from build123d import *

# Parameters (mm, degrees)
SKETCH_1_W      = 4
SKETCH_1_H      = 1
SKETCH_1_W_2    = 1
SKETCH_1_H_2    = 4
EXTRUDE_1_DEPTH = 8
CHAMFER_1_SIZE  = 0.5
CHAMFER_2_SIZE  = 0.5
SKETCH_2_R      = 7.5
EXTRUDE_2_DEPTH = 2
FILLET_1_R      = 1


# Some blends are built 0.0001 mm under size
with BuildPart() as part:
    # 草图1 → 凸台-拉伸1 (new body)
    with BuildSketch(Plane.XY):
        Rectangle(SKETCH_1_W, SKETCH_1_H)
        Rectangle(SKETCH_1_W_2, SKETCH_1_H_2)
    extrude(amount=EXTRUDE_1_DEPTH)

    # 倒角1
    chamfer_1_edges = [part.edges().sort_by_distance(p)[0] for p in [
        (-1.25, -0.5, 8),
        (-0.5, -1.25, 8),
        (0.5, -1.25, 8),
        (1.25, -0.5, 8),
        (-1.25, 0.5, 8),
        (-0.5, 1.25, 8),
        (1.25, 0.5, 8),
        (0.5, 1.25, 8),
    ]]
    chamfer(chamfer_1_edges, length=CHAMFER_1_SIZE - 0.0001)  # a hair under: the kernel refuses the full size

    # 倒角2
    # the kernel refuses this chamfer: 0.5 mm, written as the material it takes off along each edge
    with BuildSketch(Plane(origin=(-2, 1.40922724, 6.59087276), x_dir=(0.9996219169112968, 0.01944252080601401, 0.019442520806014003), z_dir=(0, -0.7071067811865474, 0.7071067811865477)), Plane(origin=(0.90912724, -2, 8.90922724), x_dir=(0.7068394360706737, -0.02749587661058652, -0.7068394360706732), z_dir=(-0.7071067811865474, 0, -0.7071067811865477)), Plane(origin=(2, 0.90912724, 8.90922724), x_dir=(0.027495876610586514, 0.7068394360706736, -0.7068394360706733), z_dir=(0, -0.7071067811865474, -0.7071067811865477)), Plane(origin=(-0.90912724, 2, 8.90922724), x_dir=(-0.7068394360706737, 0.02749587661058652, -0.7068394360706732), z_dir=(0.7071067811865474, 0, -0.7071067811865477)), Plane(origin=(-1.40922724, 2, 6.59087276), x_dir=(0.7068394360706737, 0.027495876610586494, -0.7068394360706733), z_dir=(0.7071067811865474, 0, 0.7071067811865477))) as chamfer_2_piece_1:
        Polygon((CHAMFER_2_SIZE * 0.999621916911, -CHAMFER_2_SIZE * 0.0274958766106), (-CHAMFER_2_SIZE * 0.0274958766106, -CHAMFER_2_SIZE * 0.999621916911), (0, 0), align=None)
    extrude(amount=3.278648348, mode=Mode.SUBTRACT)
    with BuildSketch(Plane(origin=(-2, 0.90912724, 8.90922724), x_dir=(-0.027495876610586514, 0.7068394360706736, -0.7068394360706733), z_dir=(0, -0.7071067811865474, -0.7071067811865477)), Plane(origin=(-0.90912724, -2, 8.90922724), x_dir=(-0.7068394360706737, -0.02749587661058652, -0.7068394360706732), z_dir=(0.7071067811865474, 0, -0.7071067811865477)), Plane(origin=(2, -0.90912724, 8.90922724), x_dir=(0.027495876610586514, -0.7068394360706736, -0.7068394360706733), z_dir=(0, 0.7071067811865474, -0.7071067811865477))) as chamfer_2_piece_2:
        Polygon((CHAMFER_2_SIZE * 0.999621916911, CHAMFER_2_SIZE * 0.0274958766106), (-CHAMFER_2_SIZE * 0.0274958766106, CHAMFER_2_SIZE * 0.999621916911), (0, 0), align=None)
    extrude(amount=3.278648348, mode=Mode.SUBTRACT)

    # 草图2 → 凸台-拉伸2 (add)
    with BuildSketch(Plane(origin=(0, 0, 0), x_dir=(-1, 0, 0), z_dir=(0, 0, -1))):
        Circle(SKETCH_2_R)
    extrude(amount=EXTRUDE_2_DEPTH)

    # 圆角1
    fillet_1_edges = [part.edges().sort_by_distance(p)[0] for p in [
        (7.5, 0, 0),
        (7.5, 0, -2),
    ]]
    fillet(fillet_1_edges, radius=FILLET_1_R - 0.0001)  # a hair under: the kernel refuses the full size


solid = part.part
CAD build for the part. Positions are in the model's coordinates, mm. A direction names the side the tool comes from. Round coordinates to 2 decimals unless told otherwise and drop trailing zeros. Order: outer loops, then holes, each group sorted by start corner. A loop starts at its lowest first (then second) coordinate and runs counter-clockwise, first axis right, second up. Notation, with made-up numbers: (71, -28) -> (114, -28) arc R30 ccw to (114, 3) -> close; hole circle Ø10 at (0.25, 66). An arc over 180 degrees is marked (long way). Write each question's results on one line, items separated by ' | '.
1. Cut at A-A (z = 2.75). Give the cut face in (x, y), plus the area to 3 significant figures.
Findings below:
outline: (-2, -0.5) -> (-0.5, -0.5) -> (-0.5, -2) -> (0.5, -2) -> (0.5, -0.5) -> (2, -0.5) -> (2, 0.5) -> (0.5, 0.5) -> (0.5, 2) -> (-0.5, 2) -> (-0.5, 0.5) -> (-2, 0.5) -> close | area: 7.00 mm²
2. 3-axis set-ups, long thin cutter, end or side, ignore diameter. For faces 1 (the face through (2, 0, 4)), 2 (the face through (0, -2, 4)), 3 (the face through (0, 2, 4)), 4 (the face through (-0.5, -1, 4)), 5 (the face through (1, 0.5, 4)): which of +Z, -Z, +X, -X, +Y, -Y reach the whole face in a straight line?
Findings below:
face 1: +Z, +X, +Y, -Y | face 2: +Z, +X, -X, -Y | face 3: +Z, +X, -X, +Y | face 4: +Z, -X, -Y | face 5: +Z, +X, +Y
3. Wall check: line 1 along Z through (x, y) = (-1, 5); line 2 along X through (y, z) = (-1.75, 6). Give the ranges that are in metal, low to high. Write a range as [from, to].
Findings below:
line 1: z = [-2, 0] | line 2: x = [-0.5, 0.5]
4. Flat gauge pins, fed straight in: P1, Ø1.5, axis at x = -5, y = -1, coming from the +Z side; P2, Ø0.8, axis at y = 1, z = 3.5, coming from the -X side; P3, Ø1.1, axis at x = 0, z = 4, coming from the -Y side. Where does each tip first touch, or does it go through?
Findings below:
P1: stops at z = 0 | P2: stops at x = -0.5 | P3: stops at y = -2
